Work out the finished part from the listing and answer in its coordinate system (mm). Face numbers are marked on the shaded views. A direction names the side the tool comes from. Coordinates: 2 decimals unless noted, no trailing zeros. Loops run counter-clockwise (first coordinate to the right, second up) from the corner with the lowest first, then second, coordinate; pieces in that order, holes last. Notation, with made-up numbers: (-0.5, 70) -> (48.5, 70) arc R15 cw to (48.5, 93) -> close; hole circle Ø4 at (76.25, 18). An arc over 180 degrees is marked (long way). Use a Markdown table: item, result. Add a question column.
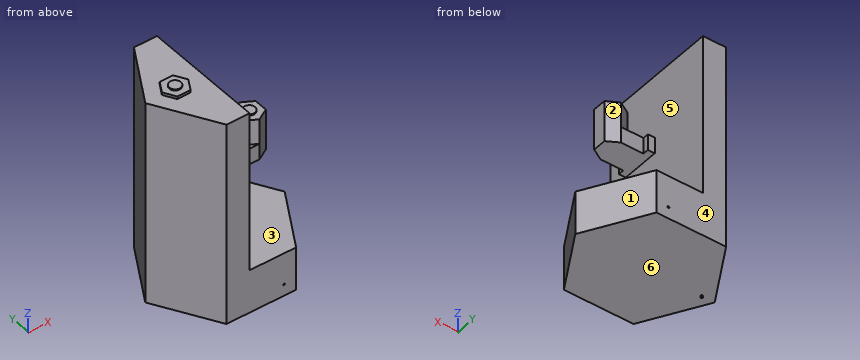
Autodesk Inventor part; units mm, degrees
ref_plane "YZ Plane" through (0, 0, 0) normal (1, 0, 0) x (0, 1, 0)
ref_plane "XZ Plane" through (0, 0, 0) normal (0, 1, 0) x (-1, 0, 0)
ref_plane "XY Plane" through (0, 0, 0) normal (0, 0, 1) x (1, 0, 0)
sketch "Sketch1" plane through (0, 0, 0) normal (0, 0, 1) x (1, 0, 0)
  line L0 (303.011, 0) -> (151.5055, -262.4152)
  line L1 (151.5055, -262.4152) -> (-151.5055, -262.4152)
  line L2 (-151.5055, -262.4152) -> (-303.011, 0)
  line L3 (-303.011, 0) -> (-151.5055, 262.4152)
  line L4 (-151.5055, 262.4152) -> (151.5055, 262.4152)
  line L5 (151.5055, 262.4152) -> (303.011, 0)
  point P0 (0, 0)
  point P1 (0, 0)
  dimension "d0" = 606.022
extrude "Extrusion1" add sketch "Sketch1" along normal blind 190.5
sketch "Sketch2" plane through (0, 0, 190.5) normal (0, 0, 1) x (1, 0, 0)
  line L0 (151.5055, -262.4152) -> (303.011, 0)
  line L1 (303.011, 0) -> (151.5055, 262.4152)
  line L2 (151.5055, 262.4152) -> (-151.5055, 262.4152) construction
  line L3 (-151.5055, 262.4152) -> (-303.011, 0)
  line L4 (-303.011, 0) -> (-151.5055, -262.4152)
  line L5 (-151.5055, -262.4152) -> (151.5055, -262.4152) construction
  line L6 (151.5055, 262.4152) -> (-151.5055, 262.4152)
  line L7 (-50.7278, 262.4152) -> (-50.7278, -262.4152)
  line L8 (-151.5055, -262.4152) -> (151.5055, -262.4152)
  line L9 (-50.7278, 262.4152) -> (-151.5055, 262.4152)
  line L10 (-50.7278, -262.4152) -> (-151.5055, -262.4152)
  point P0 (0, 0)
  dimension "d3" = 353.7388
extrude "Extrusion2" add sketch "Sketch2" along normal blind 704.85 contours L8 L4 L3 L6 L7
sketch "Sketch3" plane through (-50.7278, -262.4152, 190.5) normal (1, 0, 0) x (0, 0, -1)
  line L0 (-428.7, 86.64) -> (-358.7, 86.64)
  line L1 (-358.7, 86.64) -> (-358.7, 251.64)
  line L2 (-358.7, 251.64) -> (-428.7, 251.64)
  line L3 (-428.7, 251.64) -> (-428.7, 86.64)
  line L4 (0, 0) -> (-704.85, 0)
  line L5 (0, 0) -> (0, 262.4152)
  point P0 (190.5, 262.4152)
  dimension "d6" = 86.64
  dimension "d7" = 358.7
  dimension "d8" = 70
  dimension "d9" = 165
extrude "Extrusion3" add sketch "Sketch3" along normal blind 30
sketch "Sketch4" plane through (-20.7278, -262.4152, 190.5) normal (1, 0, 0) x (0, 0, -1)
  line L0 (-428.7, 86.64) -> (-428.7, 251.64)
  line L1 (-358.7, 251.64) -> (-358.7, 86.64)
  line L2 (-428.7, 111.64) -> (-358.7, 111.64)
  line L3 (-358.7, 111.64) -> (-358.7, 226.64)
  line L4 (-358.7, 226.64) -> (-428.7, 226.64)
  line L5 (-428.7, 226.64) -> (-428.7, 111.64)
  point P0 (190.5, 262.4152)
  point P1 (-428.7, 169.14)
  dimension "d12" = 115
extrude "Extrusion4" add sketch "Sketch4" along normal blind 98.2
sketch "Sketch5" plane through (-50.7278, -175.7752, 619.2) normal (0, 0, 1) x (1, 0, 0)
  line L0 (128.2, 25) -> (128.2, 140)
  line L1 (128.2, 140) -> (177.9965, 111.25)
  line L2 (177.9965, 111.25) -> (177.9965, 53.75)
  line L3 (177.9965, 53.75) -> (128.2, 25)
  line L4 (128.2, 25) -> (78.4035, 53.75)
  line L5 (78.4035, 53.75) -> (78.4035, 111.25)
  line L6 (78.4035, 111.25) -> (128.2, 140)
  point P0 (50.7278, 175.7752)
  point P1 (128.2, 82.5)
extrude "Extrusion5" add sketch "Sketch5" along normal blind 110 and the other way blind 70
sketch "Sketch6" plane through (0, 0, 895.35) normal (0, 0, 1) x (1, 0, 0)
  line L0 (-115.8774, 0) -> (-144.6274, -49.7965)
  line L1 (-144.6274, -49.7965) -> (-202.1274, -49.7965)
  line L2 (-202.1274, -49.7965) -> (-230.8774, 0)
  line L3 (-230.8774, 0) -> (-202.1274, 49.7965)
  line L4 (-202.1274, 49.7965) -> (-144.6274, 49.7965)
  line L5 (-144.6274, 49.7965) -> (-115.8774, 0)
  line L6 (-50.7278, -262.4152) -> (-50.7278, 262.4152)
  point P0 (0, 0)
  point P1 (-173.3774, 0)
  point P2 (-50.7278, 0)
  dimension "d19" = 115
  dimension "d20" = 122.6496
extrude "Extrusion6" add sketch "Sketch6" along normal blind 11.725
sketch "Sketch7" plane through (-50.7278, -175.7752, 729.2) normal (0, 0, 1) x (1, 0, 0)
  line L0 (177.9965, 111.25) -> (128.2, 140)
  line L1 (128.2, 140) -> (78.4035, 111.25)
  line L2 (78.4035, 111.25) -> (78.4035, 53.75)
  line L3 (78.4035, 53.75) -> (128.2, 25)
  line L4 (128.2, 25) -> (177.9965, 53.75)
  line L5 (177.9965, 53.75) -> (177.9965, 111.25)
  circle A0 centre (128.2, 82.5) radius 25
  point P0 (50.7278, 175.7752)
  point P1 (177.9965, 82.5)
  dimension "d23" = 50
extrude "Extrusion7" add sketch "Sketch7" along normal blind 5 contours A0
sketch "Sketch8" plane through (-151.5055, -262.4152, 0) normal (0, -1, 0) x (1, 0, 0)
  line L0 (303.011, 0) -> (0, 0)
  line L1 (303.011, 0) -> (303.011, 190.5)
  line L2 (100.7777, 190.5) -> (303.011, 190.5)
  line L3 (100.7777, 190.5) -> (100.7777, 895.35)
  line L4 (0, 895.35) -> (100.7777, 895.35)
  line L5 (0, 0) -> (0, 895.35)
  circle A0 centre (251.021, 50.8) radius 4
  point P0 (151.5055, 0)
  dimension "d26" = 8
  dimension "d27" = 50.8
  dimension "d28" = 51.99
extrude "Extrusion8" cut sketch "Sketch8" against normal through all contours A0
sketch "Sketch9" plane through (0, 0, 0) normal (0, 0, -1) x (-1, 0, 0)
  circle A0 centre (246.7476, 0) radius 5
  point P0 (0, 0)
  point P1 (303.011, 0)
  dimension "d31" = 10
  dimension "d32" = 56.2634
extrude "Extrusion9" add sketch "Sketch9" along normal blind 5
sketch "Sketch10" plane through (0, 0, 907.075) normal (0, 0, 1) x (1, 0, 0)
  line L0 (-144.6274, -49.7965) -> (-115.8774, 0)
  line L1 (-115.8774, 0) -> (-144.6274, 49.7965)
  line L2 (-144.6274, 49.7965) -> (-202.1274, 49.7965)
  line L3 (-202.1274, 49.7965) -> (-230.8774, 0)
  line L4 (-230.8774, 0) -> (-202.1274, -49.7965)
  line L5 (-202.1274, -49.7965) -> (-144.6274, -49.7965)
  circle A0 centre (-173.3774, 0) radius 25
  point P0 (0, 0)
  point P1 (-173.3774, 49.7965)
  dimension "d35" = 50
extrude "Extrusion10" add sketch "Sketch10" along normal blind 5 contours A0
properties material "ABS Plastic"
Item 1: Section D-D (y = 126.5) is taken. Determine the outline of the cut face in (x, z), then the cut area to 3 significant figures.
Item 2: Find the intervals of material crossed by probe 1 along Z at (x, y) = (176, -60); probe 2 along Z at (x, y) = (-126, 112); probe 3 along X at (y, z) = (105, 50), in increasing order.
Item 3: Section A-A (y = -209) is taken. Determine the outline of the cut face in (x, z), then the cut area to 3 significant figures.
Item 4: For the marked faces 1, 2 and 3, determine the directions among +Z, -Z, +X, -X, +Y, -Y from which every point of the face is accessible in a straight line to the end or side of a thin tool.
Item 5: For a pull along Z with two mould halves and no side action, classify the marked faces 4, 5 and 6 as +Z half, -Z half, draft (parallel to the pull), parting line (faces both ways), or undercut.
Item 6: Given pin 1 (1.5 mm diameter, centred on x = 109.5, y = -73.5, fed in from +Z); pin 2 (20 mm diameter, centred on y = -162.5, z = 571.5, fed in from +X); pin 3 (15 mm diameter, centred on x = -29, z = 601.5, fed in from -Y), each flat-ended and moving along its own axis, determine where each tip first touches the part or whether it passes through.
Item 7: Section C-C (z = 119.5) is taken. Determine the outline of the cut face in (x, y), then the cut area to 3 significant figures.
Item 8: Section B-B (x = 116) is taken. Determine the outline of the cut face in (y, z).
Output:
| question | item | result |
|---|---|---|
| 1 | outline | (-229.98, 0) -> (229.98, 0) -> (229.98, 190.5) -> (-50.73, 190.5) -> (-50.73, 895.35) -> (-229.98, 895.35) -> close; hole circle Ø8 at (99.52, 50.8) |
| 1 | area | 214,000 mm2 |
| 2 | probe 1 | z = 0 to 190.5 |
| 2 | probe 2 | z = 0 to 895.35 |
| 2 | probe 3 | x = -242.39 to 95.6, 103.43 to 242.39 |
| 3 | outline | (-182.34, 0) -> (182.34, 0) -> (182.34, 190.5) -> (-50.73, 190.5) -> (-50.73, 895.35) -> (-182.34, 895.35) -> close; hole circle Ø8 at (99.52, 50.8) |
| 3 | area | 162,000 mm2 |
| 4 | face 1 | +Z, -Z, +X, +Y |
| 4 | face 2 | +Z, +X, +Y |
| 4 | face 3 | +X, +Y, -Y |
| 5 | face 4 | draft |
| 5 | face 5 | undercut |
| 5 | face 6 | -Z half |
| 6 | pin 1 | stops at z = 729.2 |
| 6 | pin 2 | stops at x = -20.73 |
| 6 | pin 3 | stops at y = -175.78 |
| 7 | outline | (-303.01, 0) -> (-151.51, -262.42) -> (151.51, -262.42) -> (303.01, 0) -> (151.51, 262.42) -> (-151.51, 262.42) -> close |
| 7 | area | 239,000 mm2 |
| 8 | outline | (-262.42, 0) -> (262.42, 0) -> (262.42, 190.5) -> (-262.42, 190.5) -> close; (-128.53, 549.2) -> (-58.02, 549.2) -> (-58.02, 729.2) -> (-128.53, 729.2) -> close |
